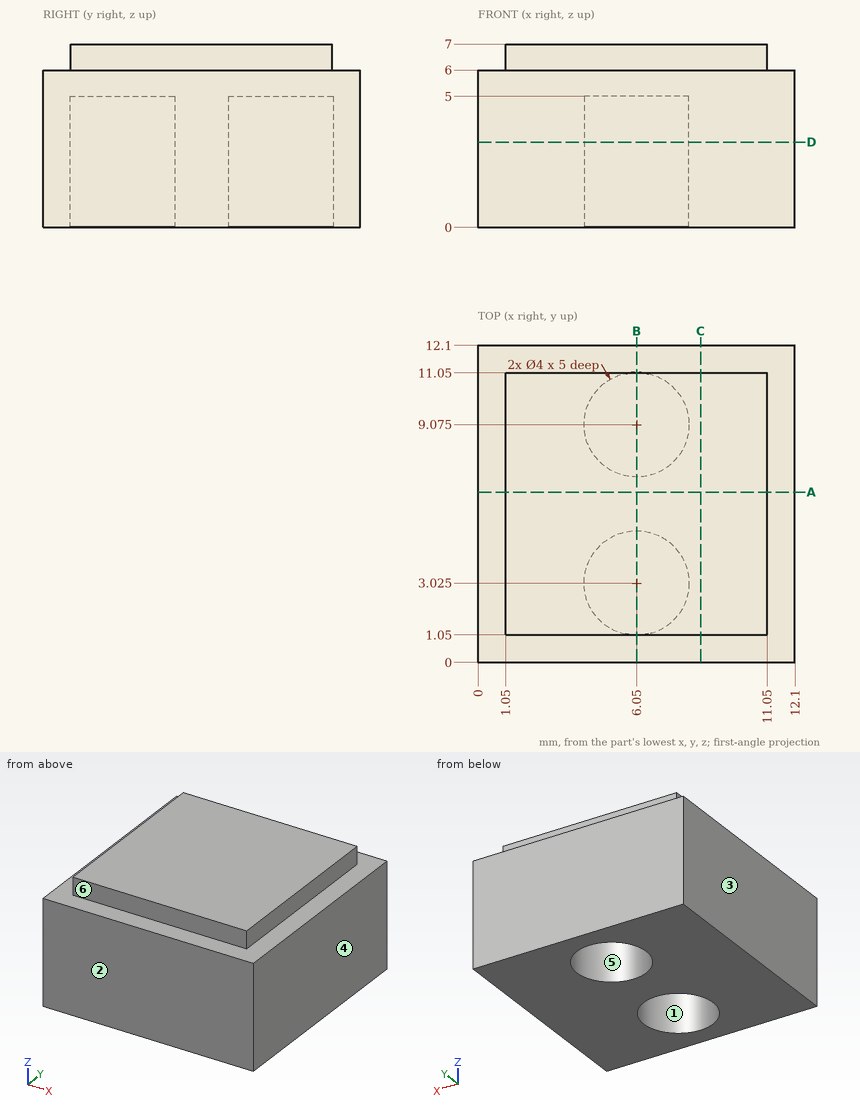
Job drawing, mm, ordinate dimensions from the low corner. One solid piece. A direction names the side the tool comes from. Coordinates: 2 decimals unless noted, no trailing zeros. Write each loop counter-clockwise with the first axis right and the second up, starting at its lowest first coordinate (ties: lowest second). Pieces come first, ordered by that corner, then holes. Notation, with made-up numbers: M 68,10 L 107,10 A34 cw 107,41 Z; hole C 79.5,59.5 d7. An arc over 180 degrees is marked long. Answer as a JSON object with one key per item and string values. Group by question number.
1) Saw through at A-A (y = 6.5). Write the cut outline in (x, z), plus the area to 3 significant figures.
2) Wall check: line 1 (Y direction, x = 6.05, z = 3.8) (3 decimals); line 2 (Y direction, x = 4.5, z = 0.75); line 3 (Z direction, x = 1, y = 2.5). Give the ranges that are in metal, low to high. Write a range as from..to.
3) Mould opens along X. For the marked faces 1, 2 and 3 say: +X half, -X half, draft (parallel to the pull), parting line (faces both ways), or undercut.
4) Saw through at D-D (z = 3.25). Write the cut outline in (x, y) (3 decimals).
5) Pin check, flat tips, straight feed: pin 1 Ø0.5 at (y, z) = (3.5, 6.5) entering from -X; pin 2 Ø1.2 at (x, y) = (5.5, 2.5) entering from -Z; pin 3 Ø0.8 at (y, z) = (8, 6.5) entering from +X. Stop position of each tip, or through.
6) Tool access for the marked faces 4, 5 and 6: list every direction of +Z, -Z, +X, -X, +Y, -Y with a clear straight run to the whole face (end or side of a thin tool).
7) Saw through at B-B (x = 6.05). Write the cut outline in (y, z) (3 decimals).
Values follow:
{
 "1": {"outline": "M 0,0 L 12.1,0 L 12.1,6 L 11.05,6 L 11.05,7 L 1.05,7 L 1.05,6 L 0,6 Z", "area": "82.6 mm2"},
 "2": {"line 1": "y = 0..1.025, 5.025..7.075, 11.075..12.1", "line 2": "y = 0..1.76, 4.29..7.81, 10.34..12.1", "line 3": "z = 0..6"},
 "3": {"face 1": "undercut", "face 2": "draft", "face 3": "-X half"},
 "4": {"outline": "M 0,0 L 12.1,0 L 12.1,12.1 L 0,12.1 Z; hole C 6.05,3.025 d4; hole C 6.05,9.075 d4"},
 "5": {"pin 1": "stops at x = 1.05", "pin 2": "stops at z = 5", "pin 3": "stops at x = 11.05"},
 "6": {"face 4": "+Z, -Z, +X, +Y, -Y", "face 5": "-Z", "face 6": "+Z, +X, -X, -Y"},
 "7": {"outline": "M 0,0 L 1.025,0 L 1.025,5 L 5.025,5 L 5.025,0 L 7.075,0 L 7.075,5 L 11.075,5 L 11.075,0 L 12.1,0 L 12.1,6 L 11.05,6 L 11.05,7 L 1.05,7 L 1.05,6 L 0,6 Z"}
}
